```python
from build123d import *

# Parameters (mm, degrees)
SKETCH1_7_W             = 89.29
SKETCH1_7_H             = 147.294272307
SKETCH1_7_R             = 1
SKETCH1_7_R_2           = 3.6
SKETCH1_7_R_3           = 3.5
BODY_DEPTH              = 3.18
SKETCH2_W               = 19.3
SKETCH2_H               = 3.18
BOSS_EXTRUDE1_DEPTH     = 3.18
SKETCH3_R               = 1.425
CUT_EXTRUDE1_DEPTH      = 89.95245291
SKETCH4_W               = 3.18
SKETCH4_H               = 19.3
BOSS_EXTRUDE2_DEPTH     = 3.18
SKETCH5_R               = 1.425
CUT_EXTRUDE2_DEPTH      = 91.482140695
MIRROR2_COPY_1_SKETCH_W = 3.18
MIRROR2_COPY_1_SKETCH_H = 19.3
MIRROR2_COPY_1_DEPTH    = 3.18
MIRROR2_COPY_2_SKETCH_R = 1.425
MIRROR2_COPY_2_DEPTH    = 91.482140695


with BuildPart() as part:
    # Sketch1_7 → Body (new body)
    with BuildSketch(Plane.XY):
        with Locations((0.105848892, -0.017058674)):
            Rectangle(SKETCH1_7_W, SKETCH1_7_H)
        with Locations(Location((-5.509858965, -44.064194828, 0), (0, 0, 180))):
            Circle(SKETCH1_7_R, mode=Mode.SUBTRACT)
        with Locations(Location((-26.900831216, -26.517202566, 0), (0, 0, 180))):
            Circle(SKETCH1_7_R_2, mode=Mode.SUBTRACT)
        with Locations(Location((-18.500240022, -51.564194828, 0), (0, 0, 180))):
            Circle(SKETCH1_7_R, mode=Mode.SUBTRACT)
        with Locations(Location((10.490141035, -44.064194828, 0), (0, 0, 180))):
            Circle(SKETCH1_7_R, mode=Mode.SUBTRACT)
        with Locations(Location((-2.500240022, -51.564194828, 0), (0, 0, 180))):
            Circle(SKETCH1_7_R, mode=Mode.SUBTRACT)
        with Locations(Location((18.957561099, -29.561304194, 0), (0, 0, 180))):
            Circle(SKETCH1_7_R_3, mode=Mode.SUBTRACT)
        with Locations(Location((33.068305831, -21.491722051, 0), (0, 0, 180))):
            Circle(SKETCH1_7_R_3, mode=Mode.SUBTRACT)
        with BuildLine():
            Line((-0.296750946, -48.342906228), (6.675853351, -44.420816311))
            ThreePointArc((6.675853351, -44.420816311), (8.847894842, -45.022980632), (8.258255476, -47.198455643))
            Line((8.258255476, -47.198455643), (1.358448729, -51.285483428))
            ThreePointArc((1.358448729, -51.285483428), (-0.940439708, -50.641794665), (-0.296750946, -48.342906228))
        make_face(mode=Mode.SUBTRACT)
        with BuildLine():
            Line((35.889642662, 62.490077479), (-35.919151108, 62.490077479))
            ThreePointArc((-35.919151108, 62.490077479), (-37.686918061, 61.757844432), (-38.419151108, 59.990077479))
            Line((-38.419151108, 59.990077479), (-38.419151108, 6.918014642))
            ThreePointArc((-38.419151108, 6.918014642), (-37.686918061, 5.150247689), (-35.919151108, 4.418014642))
            Line((-35.919151108, 4.418014642), (29.997375098, 4.418014642))
            ThreePointArc((29.997375098, 4.418014642), (35.990372343, 7.41277043), (38.389642662, 13.668014642))
            Line((38.389642662, 13.668014642), (38.389642662, 59.990077479))
            ThreePointArc((38.389642662, 59.990077479), (37.657409615, 61.757844432), (35.889642662, 62.490077479))
        make_face(mode=Mode.SUBTRACT)
        with BuildLine():
            Line((-16.296750946, -48.342906228), (-9.324146649, -44.420816311))
            ThreePointArc((-9.324146649, -44.420816311), (-7.152105158, -45.022980632), (-7.741744524, -47.198455643))
            Line((-7.741744524, -47.198455643), (-14.641551271, -51.285483428))
            ThreePointArc((-14.641551271, -51.285483428), (-16.940439708, -50.641794665), (-16.296750946, -48.342906228))
        make_face(mode=Mode.SUBTRACT)
    extrude(amount=BODY_DEPTH)

    # Sketch2 → Boss-Extrude1 (add)
    with BuildSketch(Plane(origin=(0, 73.630077479, 0), x_dir=(1, 0, 0), z_dir=(0, 1, 0))):
        with Locations((0, -1.59)):
            Rectangle(SKETCH2_W, SKETCH2_H)
    boss_extrude1 = extrude(amount=BOSS_EXTRUDE1_DEPTH)

    # Sketch3 → Cut-Extrude1 (cut, through all)
    with BuildSketch(Plane.XY.offset(3.18)):
        with Locations((0, 75.220077479)):
            Circle(SKETCH3_R)
    cut_extrude1 = extrude(amount=-CUT_EXTRUDE1_DEPTH, mode=Mode.SUBTRACT)

    # Sketch4 → Boss-Extrude2 (add)
    with BuildSketch(Plane.ZY.offset(44.539151108)):
        with Locations((1.59, 26.810077479)):
            Rectangle(SKETCH4_W, SKETCH4_H)
    boss_extrude2 = extrude(amount=BOSS_EXTRUDE2_DEPTH)

    # Sketch5 → Cut-Extrude2 (cut, through all)
    with BuildSketch(Plane.XY.offset(3.18)):
        with Locations((-46.161220751, 26.810077479)):
            Circle(SKETCH5_R)
    cut_extrude2 = extrude(amount=-CUT_EXTRUDE2_DEPTH, mode=Mode.SUBTRACT)

    # Mirror1: Boss-Extrude2, Cut-Extrude2 across plane
    add(boss_extrude2.mirror(Plane(origin=(0, 0, 0), x_dir=(0, 0, 1), z_dir=(1, 0, 0))))
    add(cut_extrude2.mirror(Plane(origin=(0, 0, 0), x_dir=(0, 0, 1), z_dir=(1, 0, 0))), mode=Mode.SUBTRACT)

    # Mirror2: Boss-Extrude1, Cut-Extrude1, Boss-Extrude2, Cut-Extrude2 across plane
    add(boss_extrude1.mirror(Plane.ZX))
    add(cut_extrude1.mirror(Plane.ZX), mode=Mode.SUBTRACT)
    add(boss_extrude2.mirror(Plane.ZX))
    add(cut_extrude2.mirror(Plane.ZX), mode=Mode.SUBTRACT)

    # Mirror2 copy 1 sketch → Mirror2 copy 1 (add)
    with BuildSketch(Plane(origin=(44.539151108, 0, 0), x_dir=(0, 0, 1), z_dir=(1, 0, 0))):
        with Locations((1.59, 26.810077479)):
            Rectangle(MIRROR2_COPY_1_SKETCH_W, MIRROR2_COPY_1_SKETCH_H)
    extrude(amount=MIRROR2_COPY_1_DEPTH)

    # Mirror2 copy 2 sketch → Mirror2 copy 2 (cut, through all)
    with BuildSketch(Plane(origin=(0, 0, 3.18), x_dir=(-1, 0, 0), z_dir=(0, 0, 1))):
        with Locations((-46.161220751, 26.810077479)):
            Circle(MIRROR2_COPY_2_SKETCH_R)
    extrude(amount=-MIRROR2_COPY_2_DEPTH, mode=Mode.SUBTRACT)


solid = part.part
```
Input: part model. Units: mm. Frame: model coordinates. A direction names the side the tool comes from. Coordinates: 2 decimals unless noted, no trailing zeros. Loops run counter-clockwise (first coordinate to the right, second up) from the corner with the lowest first, then second, coordinate; pieces in that order, holes last. Notation, with made-up numbers: M -15,52 L 27,52 A23 cw 27,75 Z; hole C 82.25,74.25 d7. An arc over 180 degrees is marked long. Use a Markdown table: item, result. Add a question column.
1) Set-up query: faces 4 (the flat face through (-27, -73.664, 2)), 5 (the flat face through (44.751, 0, 2)), 6 (the cylindrical face through (35.926, 7.342, 1.568)). Return all of +Z, -Z, +X, -X, +Y, -Y with unobstructed straight access to the full face (end or side cutting, diameter ignored); none if empty.
2) Draft query along X for faces 1 (the flat face through (-9.65, -75, 2)), 2 (the flat face through (0, -76.81, 2)), 3 (the cylindrical face through (47.212, -27.773, 1.612)). Return one class per face: +X half, -X half, draft (parallel to the pull), parting line (faces both ways), or undercut.
3) Section B-B, the plane x = -28. Return the cut outline in (y, z).
4) Section C-C, the plane y = -60. Return the cut outline in (x, z).
5) Section D-D, the plane z = 2.65. Give the number of separate pieces and of enclosed holes in the cut face, plus the area to 3 significant figures.
6) Line query: L1, parallel to Y at x = -32, z = 1.3; L2, parallel to Y at x = 3.5, z = 1.3; L3, parallel to Y at x = 10.5, z = 1.6. Output: solid intervals per line, ascending. Write a range as from..to.
7) Pin query (flat end, axial travel): P1, Ø1.6, axis at x = -46, z = 1, coming from the -Y side; P2, Ø1.6, axis at x = -13.5, z = 1, coming from the -Y side. Return the tip coordinate at first contact, or that it passes through.
8) Section A-A, the plane y = 20.5. Return the cut outline in (x, z), plus the area to 3 significant figures.
Answer below:
| question | item | result |
|---|---|---|
| 1 | face 4 | +Z, -Z, -X, -Y |
| 1 | face 5 | +Z, -Z, +X |
| 1 | face 6 | +Z, -Z |
| 2 | face 1 | -X half |
| 2 | face 2 | draft |
| 2 | face 3 | undercut |
| 3 | outline | M -73.66,0 L -29.95,0 L -29.95,3.18 L -73.66,3.18 Z; M -23.09,0 L 4.42,0 L 4.42,3.18 L -23.09,3.18 Z; M 62.49,0 L 73.63,0 L 73.63,3.18 L 62.49,3.18 Z |
| 4 | outline | M -44.54,0 L 44.75,0 L 44.75,3.18 L -44.54,3.18 Z |
| 5 | separate pieces | 1 |
| 5 | enclosed holes | 16 |
| 5 | area | 8,830 mm2 |
| 6 | L1 | -73.66..4.42, 62.49..73.63 |
| 6 | L2 | -76.81..-50.02, -46.21..4.42, 62.49..76.81 |
| 6 | L3 | -73.66..-45.06, -43.06..4.42, 62.49..73.63 |
| 7 | P1 | y = -36.46 |
| 7 | P2 | y = -73.66 |
| 8 | outline | M -47.72,0 L -38.42,0 L -38.42,3.18 L -47.72,3.18 Z; M 38.39,0 L 47.72,0 L 47.72,3.18 L 38.39,3.18 Z |
| 8 | area | 59.2 mm2 |
